For this review, take the finished solid that the model builds, in its own axes (mm). Face numbers are marked on the shaded views. A direction names the side the tool comes from. Coordinates: 2 decimals unless noted, no trailing zeros. Write each loop counter-clockwise with the first axis right and the second up, starting at its lowest first coordinate (ties: lowest second). Pieces come first, ordered by that corner, then holes. Notation, with made-up numbers: M 27.5,-19.5 L 65.5,-19.5 A35 ccw 65.5,18.5 Z; hole C 21.5,64 d3. An arc over 180 degrees is marked long. One line per question, with ' | ' between items.
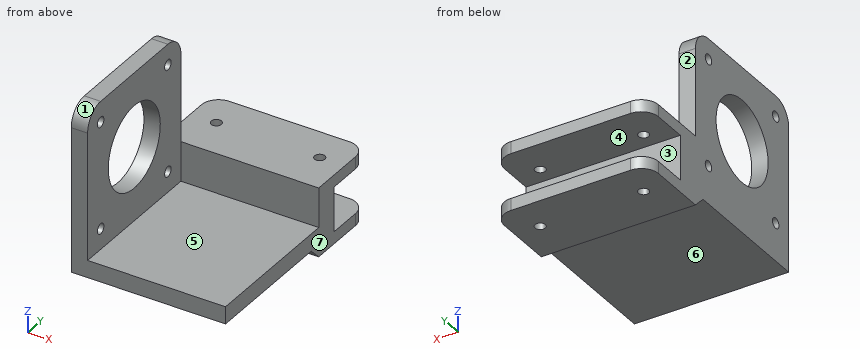
from build123d import *

# Parameters (mm, degrees)
PAD_DEPTH       = 43
SKETCH001_R     = 12
SKETCH001_R_2   = 1.5
POCKET_DEPTH    = 5
POCKET_FACE5_W  = 43
POCKET_FACE5_H  = 44.75
POCKET001_DEPTH = 15.5
SKETCH002_W     = 44.75
SKETCH002_H     = 20
PAD001_DEPTH    = 7
SKETCH003_W     = 44.75
SKETCH003_H     = 4.5
PAD002_DEPTH    = 15
SKETCH004_R     = 1.5
POCKET002_DEPTH = 20.001
CHAMFER_SIZE    = 3.49
FILLET_R        = 6
FILLET001_R     = 5
SKETCH005_W     = 48.7
SKETCH005_H     = 13
POCKET003_DEPTH = 15


with BuildPart() as part:
    # Sketch → Pad (new body)
    with BuildSketch(Plane.XZ):
        Polygon((0, 48), (0, -15.5), (44.75, -15.5), (44.75, -10.5), (4.75, -10.5), (4.75, 0), (44.75, 0), (44.75, 5), (4.75, 5), (4.75, 48), align=None)
    extrude(amount=PAD_DEPTH)

    # Sketch001 → Pocket (cut)
    with BuildSketch(Plane(origin=(4.75, 0, 0), x_dir=(0, 0, 1), z_dir=(1, 0, 0))):
        with Locations((26.5, 21.5)):
            Circle(SKETCH001_R)
        with Locations((11, 6)):
            Circle(SKETCH001_R_2)
        with Locations((11, 37)):
            Circle(SKETCH001_R_2)
        with Locations((42, 37)):
            Circle(SKETCH001_R_2)
        with Locations((42, 6)):
            Circle(SKETCH001_R_2)
    extrude(amount=-POCKET_DEPTH, mode=Mode.SUBTRACT)

    # Pocket Face5 → Pocket001 (cut)
    with BuildSketch(Plane(origin=(22.375, -21.5, -15.5), x_dir=(0, -1, 0), z_dir=(0, 0, -1))):
        Rectangle(POCKET_FACE5_W, POCKET_FACE5_H)
    extrude(amount=-POCKET001_DEPTH, mode=Mode.SUBTRACT)

    # Sketch002 (on Face2 of Pocket001) → Pad001 (join)
    with BuildSketch(Plane(origin=(0, 0, 0), x_dir=(1, 0, 0), z_dir=(0, 1, 0))):
        with Locations((22.375, -6.5)):
            Rectangle(SKETCH002_W, SKETCH002_H)
    extrude(amount=PAD001_DEPTH)

    # Sketch003 (on Face14 of Pad001) → Pad002 (join)
    with BuildSketch(Plane(origin=(0, 7, 0), x_dir=(1, 0, 0), z_dir=(0, 1, 0))):
        with Locations((22.375, -14.25)):
            Rectangle(SKETCH003_W, SKETCH003_H)
        with Locations((22.375, 1.25)):
            Rectangle(SKETCH003_W, SKETCH003_H)
    extrude(amount=PAD002_DEPTH)

    # Sketch004 (on Face22 of Pad002) → Pocket002 (cut, through all)
    with BuildSketch(Plane(origin=(0, 0, 16.5), x_dir=(-1, 0, 0), z_dir=(0, 0, 1))):
        with Locations((-37.5, -12)):
            Circle(SKETCH004_R)
        with Locations((-7.5, -12)):
            Circle(SKETCH004_R)
    extrude(amount=-POCKET002_DEPTH, mode=Mode.SUBTRACT)

    # Chamfer
    chamfer_edges = [part.edges().sort_by_distance(p)[0] for p in [
        (22.375, 0, 0),
    ]]
    chamfer(chamfer_edges, length=CHAMFER_SIZE)

    # Fillet
    fillet_edges = [part.edges().sort_by_distance(p)[0] for p in [
        (2.375, -43, 48),
        (2.375, 0, 48),
    ]]
    fillet(fillet_edges, radius=FILLET_R)

    # Fillet001
    fillet001_edges = [part.edges().sort_by_distance(p)[0] for p in [
        (0, 22, 14.25),
        (0, 22, -1.25),
        (44.75, 22, 14.25),
        (44.75, 22, -1.25),
    ]]
    fillet(fillet001_edges, radius=FILLET001_R)

    # Sketch005 (on Face28 of Fillet001) → Pocket003 (cut)
    with BuildSketch(Plane(origin=(0, 22, 0), x_dir=(1, 0, 0), z_dir=(0, 1, 0))):
        with Locations((24.35, -6.5)):
            Rectangle(SKETCH005_W, SKETCH005_H)
    extrude(amount=-POCKET003_DEPTH, mode=Mode.SUBTRACT)


solid = part.part
1) Machinability: for the marked faces 4, 5, 6 and 7, which of the approach directions +Z, -Z, +X, -X, +Y, -Y give a long, thin tool a straight path to every point of the face, cutting with its end or side? Answer none if there is none.
Responses:
face 4: +X, -X, +Y | face 5: +Z, +X, -Y | face 6: -Z, +X, -X, -Y | face 7: +Z, -Z, +X, +Y, -Y
2) The part is to be moulded in two halves that separate along Z. For the marked faces 1, 2 and 3, say which applies: +Z half, -Z half, draft (parallel to the pull), parting line (faces both ways), or undercut.
Responses:
face 1: +Z half | face 2: draft | face 3: undercut
3) We need section A-A on z = 11. State the section outline as (x, y) points.
Responses:
outline: M 0,-43 L 4.75,-43 L 4.75,-38.5 L 0,-38.5 Z; M 0,-35.5 L 4.75,-35.5 L 4.75,-7.5 L 0,-7.5 Z; M 0,-4.5 L 4.75,-4.5 L 4.75,0 L 44.75,0 L 44.75,7 L 0,7 Z
4) Insertion check: pin 1 Ø12 at (x, y) = (30.5, -14.5) entering from -Z; pin 2 Ø1 at (x, y) = (10.5, 15) entering from +Z; pin 3 Ø6 at (y, z) = (-2, 9) entering from +X; pin 4 Ø8 at (x, z) = (26.5, 16.5) entering from -Y. Each pin has a flat end and moves straight along its axis. Give the tip position at first contact, or say it passes through.
Responses:
pin 1: z = 0 | pin 2: z = 16.5 | pin 3: x = 44.75 | pin 4: y = 0
5) We need section B-B on z = 26.5. State the section outline as (x, y) points.
Responses:
outline: M 0,-43 L 4.75,-43 L 4.75,-33.5 L 0,-33.5 Z; M 0,-9.5 L 4.75,-9.5 L 4.75,0 L 0,0 Z
6) We need section C-C on y = -21.5. State the section outline as (x, z) points.
Responses:
outline: M 0,0 L 44.75,0 L 44.75,5 L 4.75,5 L 4.75,14.5 L 0,14.5 Z; M 0,38.5 L 4.75,38.5 L 4.75,48 L 0,48 Z
7) To check wall thickness, follow line 1 along Y through (x, z) = (1.6, 42); line 2 along X through (y, z) = (12, 14); line 3 along Z through (x, y) = (3, -21). State the ranges of each line that lie inside material, in increasing order. Write a range as [from, to].
Responses:
line 1: [-43, -38.5], [-35.5, -7.5], [-4.5, 0] | line 2: [0, 6], [9, 36], [39, 44.75] | line 3: [0, 14.51], [38.49, 48]
